from build123d import *

# Parameters (mm, degrees)
SKETCH1_W           = 2.7
SKETCH1_H           = 12
BOSS_EXTRUDE1_DEPTH = 0.2
CUT_EXTRUDE1_DEPTH  = 1.2
BOSS_EXTRUDE2_START = -0.55
BOSS_EXTRUDE2_DEPTH = 1.1


with BuildPart() as part:
    # Sketch1 → Boss-Extrude1 (new body)
    with BuildSketch(Plane(origin=(0, 0, 0), x_dir=(1, 0, 0), z_dir=(0, 1, 0))):
        Rectangle(SKETCH1_W, SKETCH1_H)
    extrude(amount=BOSS_EXTRUDE1_DEPTH)

    # Sketch2 → Cut-Extrude1 (cut, through all)
    with BuildSketch(Plane(origin=(0, 0, 0), x_dir=(1, 0, 0), z_dir=(0, 1, 0))):
        with BuildLine():
            Line((-1.05, 4.5), (-1.05, -4.5))
            Line((-1.05, -4.5), (1.05, -4.5))
            Line((1.05, -4.5), (1.05, 4.5))
            ThreePointArc((1.05, 4.5), (0.976776695, 4.676776695), (0.8, 4.75))
            Line((0.8, 4.75), (-0.8, 4.75))
            ThreePointArc((-0.8, 4.75), (-0.976776695, 4.676776695), (-1.05, 4.5))
        make_face()
    extrude(amount=CUT_EXTRUDE1_DEPTH, mode=Mode.SUBTRACT)

    # Sketch3 → Boss-Extrude2 (add)
    with BuildSketch(Plane(origin=(0, 0, 0), x_dir=(0, 0, -1), z_dir=(1, 0, 0)).offset(BOSS_EXTRUDE2_START)):
        with BuildLine():
            Line((4.75, 0), (4.75, 0.2))
            ThreePointArc((4.75, 0.2), (4.328691756, 0.222249459), (3.912070453, 0.288750318))
            Line((3.912070453, 0.288750318), (-1.684784687, 1.487796831))
            ThreePointArc((-1.684784687, 1.487796831), (-2.145782864, 1.377708091), (-2.35, 0.95))
            Line((-2.35, 0.95), (-2.15, 0.95))
            ThreePointArc((-2.15, 0.95), (-2.020043641, 1.222177876), (-1.726681165, 1.292234347))
            Line((-1.726681165, 1.292234347), (3.870173975, 0.093187834))
            ThreePointArc((3.870173975, 0.093187834), (4.307626344, 0.023361932), (4.75, 0))
        make_face()
    extrude(amount=BOSS_EXTRUDE2_DEPTH)


solid = part.part
Verification items for the finished model (mm, model axes). A direction names the side the tool comes from. Give positions to 0.01 mm unless a question says otherwise; leave off trailing zeros. Loops run counter-clockwise (first coordinate to the right, second up) from the corner with the lowest first, then second, coordinate; pieces in that order, holes last.
1. Cross-section at C-C on z = -0.75. Record the cut outline in (x, y).
Derived:
outline: (-1.35, 0) - (-1.05, 0) - (-1.05, 0.2) - (-1.35, 0.2) - close; (-0.55, 0.76) - (0.55, 0.76) - (0.55, 0.97) - (-0.55, 0.97) - close; (1.05, 0) - (1.35, 0) - (1.35, 0.2) - (1.05, 0.2) - close
2. Tool access check on faces 1 (the flat face through (-0.01, 0.88, -1.15)), 2 (the cylindrical face through (-0.008, 0.024, -4.301)). Record the directions out of +Z, -Z, +X, -X, +Y, -Y that give a thin tool (end or side, any length) a straight path to the whole face; none if there is none.
Derived:
face 1: -Z, +X, -X, +Y
face 2: -Y
3. Cross-section at D-D on x = 0.2. Record the cut outline in (y, z).
Derived:
outline: (0, -6) - (0.2, -6) - (0.2, -4.75) arc R4 cw to (0.29, -3.91) - (1.49, 1.68) arc R0.55 ccw to (0.95, 2.35) - (0.95, 2.15) arc R0.35 cw to (1.29, 1.73) - (0.09, -3.87) arc R4.2 ccw to (0, -4.75) - close; (0, 4.5) - (0.2, 4.5) - (0.2, 6) - (0, 6) - close
4. Cross-section at B-B on y = 1.15. Record the cut outline in (x, z), and give its area (3 significant figures).
Derived:
outline: (-0.55, 0.11) - (0.55, 0.11) - (0.55, 1.06) - (-0.55, 1.06) - close; (-0.55, 2.09) - (0.55, 2.09) - (0.55, 2.31) - (-0.55, 2.31) - close
area: 1.30 mm2
5. Release check for a two-part mould opening along Z. For faces 3 (the flat face through (-0.01, 0.7, -1.03)), 4 (the cylindrical face through (-0.008, 0.222, -4.335)) record: +Z half, -Z half, draft (parallel to the pull), parting line (faces both ways), or undercut.
Derived:
face 3: undercut
face 4: -Z half
6. Cross-section at A-A on x = 0.7. Record the cut outline in (y, z), and give its area (3 significant figures).
Derived:
outline: (0, -6) - (0.2, -6) - (0.2, -4.75) - (0, -4.75) - close; (0, 4.5) - (0.2, 4.5) - (0.2, 6) - (0, 6) - close
area: 0.550 mm2
7. Material ranges on probe 1 along X at (y, z) = (0.1, 0.5); probe 2 along Y at (x, z) = (0.3, 5.5); probe 3 along X at (y, z) = (1.35, 2), recorded low to high.
Derived:
probe 1: x = -1.35 to -1.05, 1.05 to 1.35
probe 2: y = 0 to 0.2
probe 3: x = -0.55 to 0.55
8. Go/stop test with a flat-tipped pin: P1, Ø0.8, axis at x = 0.5, z = -0.5, coming from the +Y side. Record where the tip stops, or that it passes through.
Derived:
P1: stops at y = 1.11
